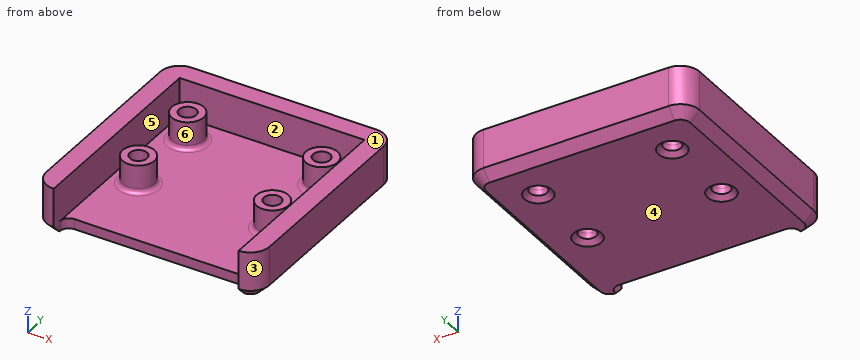
from build123d import *

# Parameters (mm, degrees)
BOSS_EXTRUDE1_DEPTH                               = 1.6
BOSS_EXTRUDE2_START                               = 6
BOSS_EXTRUDE2_DEPTH                               = 6
CSK_FOR_2_FLAT_HEAD_MACHINE_SCREW_100_D           = 2.7051
CSK_FOR_2_FLAT_HEAD_MACHINE_SCREW_100_CSINK_D     = 4.3688
CSK_FOR_2_FLAT_HEAD_MACHINE_SCREW_100_CSINK_ANGLE = 100
BOSS_EXTRUDE3_START                               = 4.35
SKETCH7_R                                         = 2.5
SKETCH7_R_2                                       = 1.35255
BOSS_EXTRUDE3_DEPTH                               = 4.35
FILLET1_R                                         = 0.7
FILLET3_R                                         = 1.4
CHAMFER1_SIZE                                     = 1.5


with BuildPart() as part:
    # Sketch1 → Boss-Extrude1 (new body)
    with BuildSketch(Plane.XY):
        with BuildLine():
            Line((-17.5, 14.5), (-17.5, -14.5))
            ThreePointArc((-17.5, -14.5), (-16.621320344, -16.621320344), (-14.5, -17.5))
            Line((-14.5, -17.5), (-14.5, -14.5))
            Line((-14.5, -14.5), (14.5, -14.5))
            Line((14.5, -14.5), (14.5, -17.5))
            ThreePointArc((14.5, -17.5), (16.621320344, -16.621320344), (17.5, -14.5))
            Line((17.5, -14.5), (17.5, 14.5))
            ThreePointArc((17.5, 14.5), (16.621320344, 16.621320344), (14.5, 17.5))
            Line((14.5, 17.5), (-14.5, 17.5))
            ThreePointArc((-14.5, 17.5), (-16.621320344, 16.621320344), (-17.5, 14.5))
        make_face()
    extrude(amount=-BOSS_EXTRUDE1_DEPTH)

    # Sketch1<3> → Boss-Extrude2 (add)
    with BuildSketch(Plane.XY.offset(BOSS_EXTRUDE2_START)):
        with BuildLine():
            ThreePointArc((-17.5, 14.5), (-16.621320344, 16.621320344), (-14.5, 17.5))
            Line((-14.5, 17.5), (14.5, 17.5))
            ThreePointArc((14.5, 17.5), (16.621320344, 16.621320344), (17.5, 14.5))
            Line((17.5, 14.5), (17.5, -14.5))
            ThreePointArc((17.5, -14.5), (16.621320344, -16.621320344), (14.5, -17.5))
            Line((14.5, -17.5), (14.5, -14.5))
            Line((14.5, -14.5), (14.5, 14.5))
            Line((14.5, 14.5), (-14.5, 14.5))
            Line((-14.5, 14.5), (-14.5, -14.5))
            Line((-14.5, -14.5), (-14.5, -17.5))
            ThreePointArc((-14.5, -17.5), (-16.621320344, -16.621320344), (-17.5, -14.5))
            Line((-17.5, -14.5), (-17.5, 14.5))
        make_face()
    extrude(amount=-BOSS_EXTRUDE2_DEPTH)

    # CSK for #2 Flat Head Machine Screw (100)1 (through all)
    with Locations(Plane(origin=(0, 0, -1.6), x_dir=(-1, 0, 0), z_dir=(0, 0, -1))):
        with Locations((10.5, 10.08), (10.5, -2.42), (-10.5, 10.08), (-10.5, -2.42)):
            CounterSinkHole(CSK_FOR_2_FLAT_HEAD_MACHINE_SCREW_100_D / 2, CSK_FOR_2_FLAT_HEAD_MACHINE_SCREW_100_CSINK_D / 2, counter_sink_angle=CSK_FOR_2_FLAT_HEAD_MACHINE_SCREW_100_CSINK_ANGLE)

    # Sketch7 → Boss-Extrude3 (add)
    # profile 1 of 4: a face of its own
    with BuildSketch(Plane.XY.offset(BOSS_EXTRUDE3_START)):
        with Locations((-10.5, 10.08)):
            Circle(SKETCH7_R)
        with Locations(Location((-10.5, 10.08, 0), (0, 0, 180))):
            Circle(SKETCH7_R_2, mode=Mode.SUBTRACT)
    # profile 2 of 4: a face of its own
    with BuildSketch(Plane.XY.offset(BOSS_EXTRUDE3_START)):
        with Locations((10.5, 10.08)):
            Circle(SKETCH7_R)
        with Locations(Location((10.5, 10.08, 0), (0, 0, 180))):
            Circle(SKETCH7_R_2, mode=Mode.SUBTRACT)
    # profile 3 of 4: a face of its own
    with BuildSketch(Plane.XY.offset(BOSS_EXTRUDE3_START)):
        with Locations((10.5, -2.42)):
            Circle(SKETCH7_R)
        with Locations(Location((10.5, -2.42, 0), (0, 0, 180))):
            Circle(SKETCH7_R_2, mode=Mode.SUBTRACT)
    # profile 4 of 4: a face of its own
    with BuildSketch(Plane.XY.offset(BOSS_EXTRUDE3_START)):
        with Locations((-10.5, -2.42)):
            Circle(SKETCH7_R)
        with Locations(Location((-10.5, -2.42, 0), (0, 0, 180))):
            Circle(SKETCH7_R_2, mode=Mode.SUBTRACT)
    extrude(amount=-BOSS_EXTRUDE3_DEPTH)

    # Fillet1
    fillet1_edges = [part.edges().sort_by_distance(p)[0] for p in [
        (8, -2.42, 0),
        (-13, -2.42, 0),
        (-13, 10.08, 0),
        (8, 10.08, 0),
    ]]
    fillet(fillet1_edges, radius=FILLET1_R)

    # Fillet3
    fillet3_edges = [part.edges().sort_by_distance(p)[0] for p in [
        (14.5, -14.5, -0.8),
        (-14.5, -14.5, -0.8),
    ]]
    fillet(fillet3_edges, radius=FILLET3_R)

    # Chamfer1
    chamfer1_edges = [part.edges().sort_by_distance(p)[0] for p in [
        (16.621320344, -16.621320344, -1.6),
        (17.5, 0, -1.6),
        (16.621320344, 16.621320344, -1.6),
        (0, 17.5, -1.6),
        (-16.621320344, 16.621320344, -1.6),
        (-17.5, 0, -1.6),
        (-16.621320344, -16.621320344, -1.6),
    ]]
    chamfer(chamfer1_edges, length=CHAMFER1_SIZE)


solid = part.part
Source: CAD feature listing. Evaluate the final solid. Frame: model axes, mm. Face numbers are marked on the shaded views. A direction names the side the tool comes from. Coordinates: 2 decimals unless noted, no trailing zeros. Write each loop counter-clockwise with the first axis right and the second up, starting at its lowest first coordinate (ties: lowest second). Pieces come first, ordered by that corner, then holes. Notation, with made-up numbers: M -10.5,-23 L 12.5,-23 A31 cw 12.5,6 Z; hole C 19,-12 d9. An arc over 180 degrees is marked long. Use a Markdown table: item, result.
1) First-contact query: pin 1 Ø8 at (x, y) = (-11, 9) entering from -Z; pin 2 Ø3 at (x, y) = (-10.5, 10.08) entering from -Z; pin 3 Ø8.5 at (x, y) = (1.5, -2.5) entering from +Z; pin 4 Ø2.5 at (x, y) = (11.5, 11) entering from +Z. Flat tips, straight axial feed; report the tip coordinate or a pass-through.
Conclusion:
| item | result |
|---|---|
| pin 1 | stops at z = -1.6 |
| pin 2 | stops at z = -1.03 |
| pin 3 | stops at z = 0 |
| pin 4 | stops at z = 4.35 |
2) Reachability of the marked faces 4, 5 and 6 from +Z, -Z, +X, -X, +Y, -Y: full face, straight path, thin tool, end or side. Return the list, or none.
Conclusion:
| item | result |
|---|---|
| face 4 | -Z, +X, -X, +Y, -Y |
| face 5 | +Z, -Y |
| face 6 | +Z |
3) Mould query, pull axis Y, two halves, no side actions, for the marked faces 1, 2 and 3. Classes: pulls with the +Y half, pulls with the -Y half, needs draft (parallel to the pull), parting line crosses it, or undercut.
Conclusion:
| item | result |
|---|---|
| face 1 | needs draft |
| face 2 | undercut |
| face 3 | pulls with the -Y half |
4) Section D-D, the plane y = 3. Output: boundary loops of the cut face in (x, z).
Conclusion:
| item | result |
|---|---|
| outline | M -17.5,-0.1 L -16,-1.6 L 16,-1.6 L 17.5,-0.1 L 17.5,6 L 14.5,6 L 14.5,0 L -14.5,0 L -14.5,6 L -17.5,6 Z |
5) Section A-A, the plane z = 1.25. Give the number of separate pieces and of enclosed holes in the cut face, then the cut area to 3 significant figures.
Conclusion:
| item | result |
|---|---|
| separate pieces | 5 |
| enclosed holes | 4 |
| area | 345 mm^2 |
6) Ray query, L1, parallel to X at y = -11.5, z = 2.5; L2, parallel to Y at x = 10.5, z = -0.6; L3, parallel to X at y = -2.42, z = -0.6. Return the intervals inside material, ascending.
Conclusion:
| item | result |
|---|---|
| L1 | x = -17.5 to -14.5, 14.5 to 17.5 |
| L2 | y = -14.5 to -3.77, -1.07 to 8.73, 11.43 to 17 |
| L3 | x = -17 to -11.85, -9.15 to 9.15, 11.85 to 17 |
